Study the drawing (mm; zero at the part's minimum x, y, z) and answer. Round coordinates to 2 decimals unless told otherwise and drop trailing zeros. Loops run counter-clockwise (first coordinate to the right, second up) from the corner with the lowest first, then second, coordinate; pieces in that order, holes last. Notation, with made-up numbers: (48.5, 79) - (64.5, 79) arc R23 ccw to (64.5, 104) - close; hole circle Ø3 at (0, -32). An arc over 180 degrees is marked (long way). Use CSV: the item, a comma, the result in double quotes. Start each with the question number.
1. Find section B-B (x = 44.45). Give the vertices of the cut face in (y, z).
2. Determine the mould class of the marked faces 1, 2 and 3 for opening direction Y: +Y half, -Y half, draft (parallel to the pull), parting line (faces both ways), or undercut.
3. Consider line 1 along Y through (x, z) = (44.45, 4.75); line 2 along Y through (x, z) = (19.05, 4) (1 decimal); line 3 along X through (y, z) = (5, 10.75) (1 decimal). Determine where each line is inside the solid, lowest interval first.
4. Find section D-D (z = 3.5). State how many separate pieces and enclosed holes the cut face has, and give its area (3 significant figures).
5. Find section C-C (y = 44.45). Give the vertices of the cut face in (x, z).
6. Find section A-A (y = 25.4). Give the vertices of the cut face in (x, z).
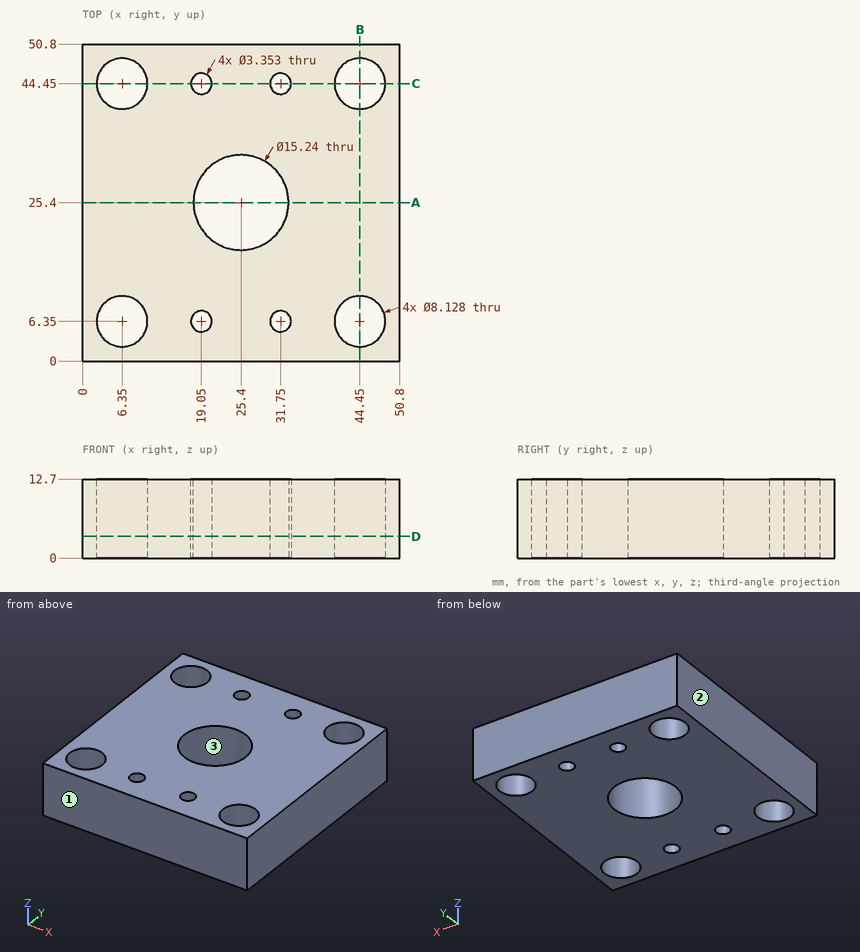
Filled sheet:
1,outline,"(0, 0) - (2.29, 0) - (2.29, 12.7) - (0, 12.7) - close; (10.41, 0) - (40.39, 0) - (40.39, 12.7) - (10.41, 12.7) - close; (48.51, 0) - (50.8, 0) - (50.8, 12.7) - (48.51, 12.7) - close"
2,face 1,"-Y half"
2,face 2,"draft"
2,face 3,"undercut"
3,line 1,"y = 0 to 2.29, 10.41 to 40.39, 48.51 to 50.8"
3,line 2,"y = 0 to 4.7, 8 to 21.2, 29.6 to 42.8, 46.1 to 50.8"
3,line 3,"x = 0 to 2.5, 10.2 to 18.1, 20 to 30.8, 32.7 to 40.6, 48.3 to 50.8"
4,separate pieces,"1"
4,enclosed holes,"9"
4,area,"2,160 mm²"
5,outline,"(0, 0) - (2.29, 0) - (2.29, 12.7) - (0, 12.7) - close; (10.41, 0) - (17.37, 0) - (17.37, 12.7) - (10.41, 12.7) - close; (20.73, 0) - (30.07, 0) - (30.07, 12.7) - (20.73, 12.7) - close; (33.43, 0) - (40.39, 0) - (40.39, 12.7) - (33.43, 12.7) - close; (48.51, 0) - (50.8, 0) - (50.8, 12.7) - (48.51, 12.7) - close"
6,outline,"(0, 0) - (17.78, 0) - (17.78, 12.7) - (0, 12.7) - close; (33.02, 0) - (50.8, 0) - (50.8, 12.7) - (33.02, 12.7) - close"
